Can you work these out from the model? Positions are in its coordinate system, mm. Face numbers are marked on the shaded views. A direction names the side the tool comes from. Coordinates: 2 decimals unless noted, no trailing zeros. Write each loop counter-clockwise with the first axis right and the second up, starting at its lowest first coordinate (ties: lowest second). Pieces come first, ordered by that corner, then holes. Notation, with made-up numbers: (-36.5, -39.75) - (-15.5, -39.75) arc R33 cw to (-15.5, -4.75) - close; hole circle Ø4 at (12.25, -23). An arc over 180 degrees is marked (long way). Use one line per item in the form item = value. Start each with the question number.
(1) On a 3-axis mill with a long thin cutter (end or side, diameter ignored), from which of +Z, -Z, +X, -X, +Y, -Y can I reach the whole of each face in a straight line? I mean the marked faces 1, 2, 3 and 4. Say none if no direction works.
(2) Thinking about a two-plate mould opening in X: for the marked faces 5, 6 and 7, which applies, pulls with the +X half, pulls with the -X half, needs draft (parallel to the pull), parting line crosses it, or undercut?
(3) If we section it at B-B on y = 13: Please give me the cut outline in (x, z), then the cut area to 3 significant figures.
(4) If we section it at C-C on x = 0: Please give me the cut outline in (y, z).
(5) If we section it at D-D on z = 6.5: Please give me the cut outline in (x, y).
(6) If I drill on probe 1 along Z at (x, y) = (0, 2.5); probe 2 along Y at (x, z) = (0.25, 14); probe 3 along X at (y, z) = (13, 5.5), over which ranges is the centre line in solid material (lowest first)? Write a range as from..to.
(7) If we section it at A-A on y = 3.5: Please give me the cut outline in (x, z).
(8) For pin 1 Ø1 at (x, z) = (3, 18.5) entering from -Y; pin 2 Ø0.6 at (x, y) = (-3, 13) entering from -Z; pin 3 Ø0.7 at (x, z) = (1.5, -3) entering from -Y; pin 4 Ø1.8 at (y, z) = (14, -1.5) entering from -X, each with a flat end and sliding along its axis, tell me the tip position at first contact or that it passes through.
```python
from build123d import *

# Parameters (mm, degrees)
SKETCH_1_R          = 3.5
EXTRUDE_1_DEPTH     = 3
EXTRUDE_2_DEPTH     = 5
SKETCH_3_R          = 2.75
EXTRUDE_3_DEPTH     = 2
SKETCH_4_R          = 2.5
CUT_EXTRUDE_1_DEPTH = 5
SKETCH_5_W          = 6
SKETCH_5_H          = 6
EXTRUDE_4_DEPTH     = 6
SKETCH_6_R          = 3.5
EXTRUDE_7_DEPTH     = 40


with BuildPart() as part:
    # 草图1 → 凸台-拉伸1 (new body)
    with BuildSketch(Plane(origin=(0, 0, 0), x_dir=(1, 0, 0), z_dir=(0, 1, 0))):
        Circle(SKETCH_1_R)
    extrude(amount=EXTRUDE_1_DEPTH)

    # 草图2 → 凸台-拉伸2 (add)
    with BuildSketch(Plane(origin=(0, 3, 0), x_dir=(1, 0, 0), z_dir=(0, 1, 0))):
        Polygon((2.642653224, 3.057730738), (-1.326745885, 3.817470195), (-3.96939911, 0.759739456), (-2.642653224, -3.057730738), (1.326745885, -3.817470195), (3.96939911, -0.759739456), align=None)
    extrude(amount=EXTRUDE_2_DEPTH)

    # 草图3 → 凸台-拉伸3 (add)
    with BuildSketch(Plane(origin=(0, 8, 0), x_dir=(1, 0, 0), z_dir=(0, 1, 0))):
        Circle(SKETCH_3_R)
    extrude(amount=EXTRUDE_3_DEPTH)

    # 草图4 → 切除-拉伸1 (cut)
    with BuildSketch(Plane.XZ):
        Circle(SKETCH_4_R)
    extrude(amount=-CUT_EXTRUDE_1_DEPTH, mode=Mode.SUBTRACT)

    # 草图5 → 凸台-拉伸4 (add)
    with BuildSketch(Plane(origin=(0, 10, 0), x_dir=(1, 0, 0), z_dir=(0, 1, 0))):
        Rectangle(SKETCH_5_W, SKETCH_5_H)
    extrude(amount=EXTRUDE_4_DEPTH)

    # 草图6 → 凸台-拉伸7 (add)
    with BuildSketch(Plane.XY.offset(3)):
        with Locations((0, 13)):
            Circle(SKETCH_6_R)
    extrude(amount=EXTRUDE_7_DEPTH)

    # 草图7 → 旋转1 (revolve)
    with BuildSketch(Plane(origin=(0, 0, 0), x_dir=(0, 0, -1), z_dir=(1, 0, 0))):
        Polygon((-43, 16.5), (-43, 13), (-45, 13), (-45, 13.5), align=None)
    revolve(axis=Axis((0, 13, 43), (0, 0, -1)))


solid = part.part
```
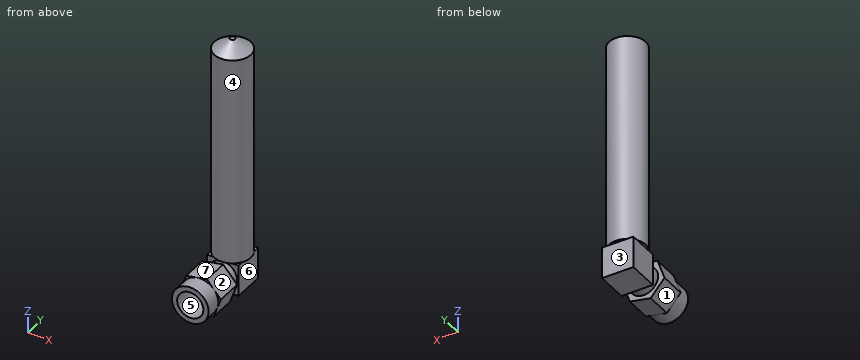
Reported:
q1.face_1 = -Z, -X, -Y
q1.face_2 = +Z, +X, -Y
q1.face_3 = -Z, +X, -X, +Y
q1.face_4 = +Z
q2.face_5 = undercut
q2.face_6 = pulls with the +X half
q2.face_7 = pulls with the -X half
q3.outline = (-3.5, 3) - (-3, 3) - (-3, -3) - (3, -3) - (3, 3) - (3.5, 3) - (3.5, 43) - (0.5, 45) - (-0.5, 45) - (-3.5, 43) - close
q3.area = 324 mm2
q4.outline = (0, -3.5) - (3, -3.5) - (3, -3.56) - (8, -3.56) - (8, -2.75) - (10, -2.75) - (10, -3) - (16, -3) - (16, 3) - (16.5, 3) - (16.5, 43) - (13.5, 45) - (12.5, 45) - (9.5, 43) - (9.5, 3) - (10, 3) - (10, 2.75) - (8, 2.75) - (8, 3.56) - (3, 3.56) - (3, 3.5) - (0, 3.5) - (0, 2.5) - (5, 2.5) - (5, -2.5) - (0, -2.5) - close
q5.outline = circle Ø7 at (0, 13)
q6.probe_1 = -3.5..-2.5, 2.5..3.5
q6.probe_2 = 9.51..16.49
q6.probe_3 = -3.5..3.5
q7.outline = (-3.97, -0.76) - (-1.33, -3.82) - (2.64, -3.06) - (3.97, 0.76) - (1.33, 3.82) - (-2.64, 3.06) - close; hole circle Ø5 at (0, 0)
q8.pin_1 = 10.55
q8.pin_2 = -3
q8.pin_3 = 0
q8.pin_4 = -3
